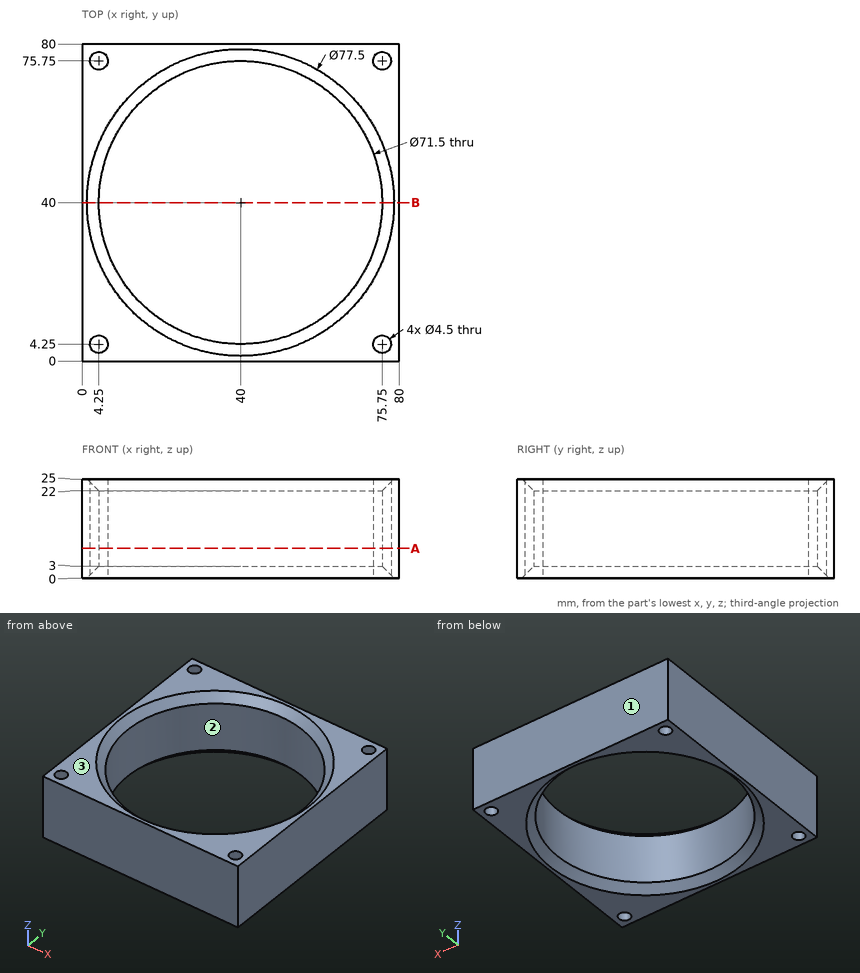
Here's the drawing with two shaded views (mm, measured from the low corner). I have some questions. Give positions to 0.01 mm unless a question says otherwise; leave off trailing zeros. Write each loop counter-clockwise with the first axis right and the second up, starting at its lowest first coordinate (ties: lowest second). Pieces come first, ordered by that corner, then holes. Notation, with made-up numbers: (77.5, 44) -> (96.5, 44) arc R30 cw to (96.5, 68) -> close; hole circle Ø9 at (46, 14). An arc over 180 degrees is marked (long way). Use one line per item in the form item = value. Start each with the question number.
1. Thinking about a two-plate mould opening in Y: for the marked faces 1, 2 and 3, which applies, +Y half, -Y half, draft (parallel to the pull), parting line (faces both ways), or undercut?
2. If I drill on L1, parallel to X at y = 39, z = 14; L2, parallel to X at y = 76.5, z = 18, over which ranges is the centre line in solid material (lowest first)?
3. Will these pins go through, and if not, where does the flat tip stop? pin 1 Ø6 at (x, y) = (4.25, 75.75) entering from -Z; pin 2 Ø8 at (x, y) = (26, 67) entering from +Z; pin 3 Ø5 at (x, y) = (21.5, 69.5) entering from +Z.
4. Imagine slicing it at B-B on y = 40. List the corners of the cut face in (x, z) for me.
5. Imagine slicing it at A-A on z = 7.5. List the corners of the cut face in (x, y) for me.
Entries:
q1.face_1 = +Y half
q1.face_2 = undercut
q1.face_3 = draft
q2.L1 = 0 to 4.26, 75.74 to 80
q2.L2 = 0 to 2.13, 6.37 to 73.63, 77.87 to 80
q3.pin_1 = 0
q3.pin_2 = through
q3.pin_3 = 23.57
q4.outline = (0, 0) -> (1.25, 0) -> (4.25, 3) -> (4.25, 22) -> (1.25, 25) -> (0, 25) -> close; (75.75, 3) -> (78.75, 0) -> (80, 0) -> (80, 25) -> (78.75, 25) -> (75.75, 22) -> close
q5.outline = (0, 0) -> (80, 0) -> (80, 80) -> (0, 80) -> close; hole circle Ø4.5 at (4.25, 4.25); hole circle Ø4.5 at (4.25, 75.75); hole circle Ø71.5 at (40, 40); hole circle Ø4.5 at (75.75, 4.25); hole circle Ø4.5 at (75.75, 75.75)
